Input: part model. Units: mm. Frame: model coordinates. A direction names the side the tool comes from. Give positions to 0.01 mm unless a question says otherwise; leave off trailing zeros. Loops run counter-clockwise (first coordinate to the right, second up) from the corner with the lowest first, then second, coordinate; pieces in that order, holes last.
from build123d import *

# Parameters (mm, degrees)
BASPROSKE_W         = 6
BASPROSKE_H         = 15
TOOTHCUT_DEPTH      = 23.045407685
TEETHCUTS_COUNT     = 18
TEETHCUTS_ANGLE     = 340
BORSKE_R            = 1.5
BORE_DEPTH          = 50.0000508
MOVE_BODY_10_ANGLE  = 10
EXTRUDE_2_DEPTH     = 6
SKETCH_2_R          = 1.65
CUT_EXTRUDE_1_DEPTH = 6
SKETCH_3_R          = 10.25
CUT_EXTRUDE_2_DEPTH = 2
FILLET_1_R          = 2


with BuildPart() as part:
    # BasProSke → Base-Revolve (revolve)
    with BuildSketch(Plane(origin=(0, 0, 0), x_dir=(1, 0, 0), z_dir=(0, 1, 0)), mode=Mode.PRIVATE) as base_revolve_sk:
        with Locations((3, 7.5)):
            Rectangle(BASPROSKE_W, BASPROSKE_H)
    revolve(base_revolve_sk.sketch.rotate(Axis((-10, 0, 0), (1, 0, 0)), 180), axis=Axis((-10, 0, 0), (1, 0, 0)))

    # TooCutSke → ToothCut (cut, through all)
    with BuildSketch(Plane(origin=(0, 0, 0), x_dir=(0, 0, -1), z_dir=(1, 0, 0))):
        with BuildLine():
            ThreePointArc((0.759974923, 11.599129886), (0, 11.624), (-0.759974923, 11.599129886))
            ThreePointArc((-0.759974923, 11.599129886), (-1.229186471, 13.354767823), (-2.254227748, 14.855339189))
            ThreePointArc((-2.254227748, 14.855339189), (0, 15.0254), (2.254227748, 14.855339189))
            ThreePointArc((2.254227748, 14.855339189), (1.229186471, 13.354767823), (0.759974923, 11.599129886))
        make_face()
    toothcut = extrude(amount=TOOTHCUT_DEPTH, mode=Mode.SUBTRACT)

    # TeethCuts: ToothCut ×18 about axis
    teethcuts_axis = Axis((-10, 0, 0), (1, 0, 0))
    for i in range(1, TEETHCUTS_COUNT):
        add(toothcut.rotate(teethcuts_axis, i * TEETHCUTS_ANGLE / (TEETHCUTS_COUNT - 1)), mode=Mode.SUBTRACT)

    # BorSke → Bore (cut, symmetric)
    with BuildSketch(Plane(origin=(0, 0, 0), x_dir=(0, 0, -1), z_dir=(1, 0, 0))):
        with Locations(Location((0, 0, 0), (0, 0, 180))):
            Circle(BORSKE_R)
    extrude(amount=BORE_DEPTH, both=True, mode=Mode.SUBTRACT)


with BuildPart() as part_1:
    # Move Body 10: moved
    add(part.part.rotate(Axis((0, 0, 0), (-1, 0, 0)), MOVE_BODY_10_ANGLE))

    # Sketch 1 → Extrude 2 (add)
    with BuildSketch(Plane(origin=(6, 0, 0), x_dir=(0, 0, -1), z_dir=(1, 0, 0))):
        Polygon((-10.545854675, -4.889000426), (-42.365659829, -36.708805579), (-42.365659829, -86.708805579), (18.256118436, -121.708805579), (18.256118436, -112.471201272), (-34.365659829, -82.090003426), (-34.365659829, -40.022514078), (-4.889000426, -10.545854675), align=None)
    extrude(amount=-EXTRUDE_2_DEPTH)

    # Sketch 2 → Cut-Extrude 1 (cut)
    with BuildSketch(Plane(origin=(6, 0, 0), x_dir=(0, 0, -1), z_dir=(1, 0, 0))):
        with Locations((-7, 0)):
            Circle(SKETCH_2_R)
        with Locations((0, 7)):
            Circle(SKETCH_2_R)
        with Locations((7, 0)):
            Circle(SKETCH_2_R)
        with Locations((0, -7)):
            Circle(SKETCH_2_R)
    extrude(amount=-CUT_EXTRUDE_1_DEPTH, mode=Mode.SUBTRACT)

    # Sketch 3 → Cut-Extrude 2 (cut)
    with BuildSketch(Plane(origin=(6, 0, 0), x_dir=(0, 0, -1), z_dir=(1, 0, 0))):
        Circle(SKETCH_3_R)
    extrude(amount=-CUT_EXTRUDE_2_DEPTH, mode=Mode.SUBTRACT)

    # Fillet 1
    fillet_1_edges = [part_1.edges().sort_by_distance(p)[0] for p in [
        (3, -121.708805579, -18.256118436),
        (3, -40.022514078, 34.365659829),
        (3, -82.090003426, 34.365659829),
    ]]
    fillet(fillet_1_edges, radius=FILLET_1_R)


solid = part_1.part
(1) Cut plane A-A (z = 28.5). Return the cut outline in (x, y), and give its area (3 significant figures).
Values follow:
outline: (0, -94.71) - (6, -94.71) - (6, -85.48) - (0, -85.48) - close; (0, -34.16) - (6, -34.16) - (6, -22.84) - (0, -22.84) - close
area: 123 mm2
(2) Ray query, probe 1 along Y at (x, z) = (5.2, 0); probe 2 along Y at (x, z) = (2.1, 7); probe 3 along Y at (x, z) = (1.2, 13). Return the intervals inside material, ascending.
Values follow:
probe 1: y = -111.17 to -101.93, -15 to -10.25, 10.25 to 15
probe 2: y = -107.13 to -97.89, -12.66 to -1.65, 1.65 to 10.32
probe 3: y = -103.66 to -94.43, -18.66 to -6.85, -3.41 to -1.08, 1.08 to 3.41, 6.85 to 7.48
(3) Cut plane B-B (y = -43.5). Return the cut outline in (x, z).
Values follow:
outline: (0, 34.37) - (6, 34.37) - (6, 42.37) - (0, 42.37) - close
(4) Cut plane C-C (x = 2.85). Count the separate pieces of the cut face and the enclosed holes in it, and give its area (3 significant figures).
Values follow:
separate pieces: 1
enclosed holes: 5
area: 1,730 mm2
(5) Reachability of faces 1 (the cylindrical face through (2.96, 1.23, 13.36)), 2 (the flat face through (4, 0, -2)), 3 (the cylindrical face through (2.96, 3.41, -12.98)), 4 (the cylindrical face through (2.958, 1.212, -13.318)) from +Z, -Z, +X, -X, +Y, -Y: full face, straight path, thin tool, end or side. Return the list, or none.
Values follow:
face 1: +Z, +X, -X
face 2: +X
face 3: +X, -X
face 4: -Z, +X, -X
(6) Pin query (flat end, axial travel): pin 1 Ø4.5 at (y, z) = (7, 0) entering from -X; pin 2 Ø3 at (x, z) = (5, 21.5) entering from +Y; pin 3 Ø1 at (x, z) = (1, 0.5) entering from -Y; pin 4 Ø4 at (y, z) = (-7, 0) entering from +X. Return the tip coordinate at first contact, or that it passes through.
Values follow:
pin 1: stops at x = 0
pin 2: stops at y = -14.34
pin 3: stops at y = -111.17
pin 4: stops at x = 4
(7) Mould query, pull axis Y, two halves, no side actions, for faces 5 (the flat face through (3.04, -103.11, 13.96)), 6 (the cylindrical face through (2.958, 12.905, 3.506)), 7 (the flat face through (3, -115, -18.256)), 8 (the cylindrical face through (2.958, -1.212, 13.318)). Classes: +Y half, -Y half, draft (parallel to the pull), parting line (faces both ways), or undercut.
Values follow:
face 5: -Y half
face 6: +Y half
face 7: draft
face 8: undercut
(8) Cut plane D-D (y = -92). Return the cut outline in (x, z).
Values follow:
outline: (0, 17.2) - (6, 17.2) - (6, 33.2) - (0, 33.2) - close
